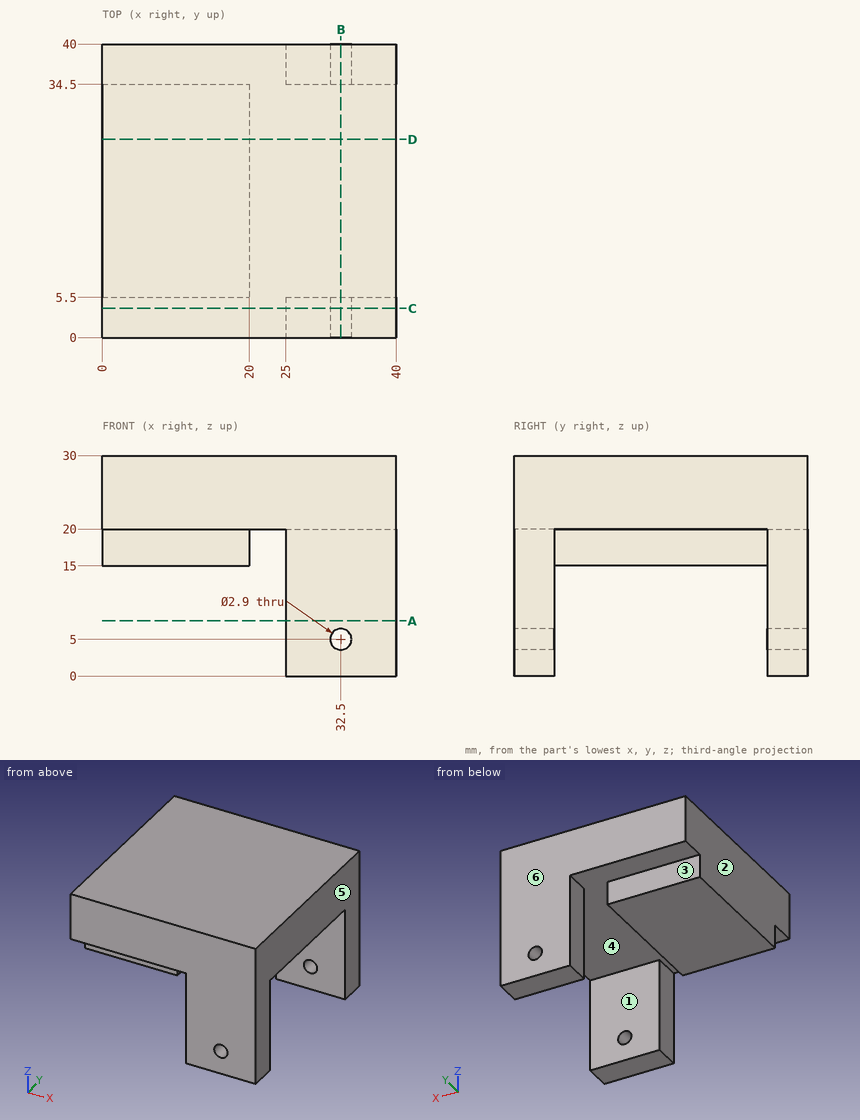
Source: three-view drawing plus pictorial views. Frame: mm from the lowest corner of the part. A direction names the side the tool comes from. Round coordinates to 2 decimals unless told otherwise and drop trailing zeros. Order: outer loops, then holes, each group sorted by start corner. A loop starts at its lowest first (then second) coordinate and runs counter-clockwise, first axis right, second up. Notation, with made-up numbers: (24.25, 62.5) -> (71.25, 62.5) arc R13 cw to (71.25, 72.5) -> close; hole circle Ø8 at (70, 39.5). An arc over 180 degrees is marked (long way). Use CSV: the item, a comma, the result in double quotes. Start each with the question number.
1) Material intervals for line 1 along Y through (x, z) = (34, 17.5); line 2 along Z through (x, y) = (32.5, 37.05); line 3 along Z through (x, y) = (27, 16.5), sorted ascending. Write a range as from..to.
2) First-contact query: pin 1 Ø6 at (y, z) = (37, 11) entering from -X; pin 2 Ø1.5 at (x, z) = (13.5, 17) entering from +Y; pin 3 Ø2.5 at (x, z) = (10.5, 16.5) entering from -Y; pin 4 Ø4 at (x, z) = (34, 13) entering from -Y. Flat tips, straight axial feed; report the tip coordinate or a pass-through.
3) Section B-B (x = 32.5). Return the cut outline in (y, z), and give its area (3 significant figures).
4) Section C-C (y = 4). Return the cut outline in (x, z).
5) Set-up query: the marked faces 1, 2 and 3. Return all of +Z, -Z, +X, -X, +Y, -Y with unobstructed straight access to the full face (end or side cutting, diameter ignored); none if empty.
6) Section D-D (y = 27). Return the cut outline in (x, z).
7) Section A-A (z = 7.5). Return the cut outline in (x, y).
8) Draft query along Y for the marked faces 4, 5 and 6. Return one class per face: +Y half, -Y half, draft (parallel to the pull), parting line (faces both ways), or undercut.
Returned:
1,line 1,"y = 0..5.5, 34.5..40"
1,line 2,"z = 0..3.55, 6.45..30"
1,line 3,"z = 20..30"
2,pin 1,"stops at x = 25"
2,pin 2,"stops at y = 34.5"
2,pin 3,"stops at y = 5.5"
2,pin 4,"stops at y = 0"
3,outline,"(0, 0) -> (5.5, 0) -> (5.5, 3.55) -> (0, 3.55) -> close; (0, 6.45) -> (5.5, 6.45) -> (5.5, 20) -> (34.5, 20) -> (34.5, 6.45) -> (40, 6.45) -> (40, 30) -> (0, 30) -> close; (34.5, 0) -> (40, 0) -> (40, 3.55) -> (34.5, 3.55) -> close"
3,area,"588 mm²"
4,outline,"(0, 20) -> (25, 20) -> (25, 0) -> (40, 0) -> (40, 30) -> (0, 30) -> close; hole circle Ø2.9 at (32.5, 5)"
5,face 1,"-Z, +X"
5,face 2,"+Z, -Z, -X, +Y, -Y"
5,face 3,"-Z, -X, +Y"
6,outline,"(0, 15) -> (20, 15) -> (20, 20) -> (40, 20) -> (40, 30) -> (0, 30) -> close"
7,outline,"(25, 0) -> (40, 0) -> (40, 5.5) -> (25, 5.5) -> close; (25, 34.5) -> (40, 34.5) -> (40, 40) -> (25, 40) -> close"
8,face 4,"undercut"
8,face 5,"draft"
8,face 6,"+Y half"
